Design review of the part built by this model. Coordinates are the model's own, in mm. Coordinates: 2 decimals unless noted, no trailing zeros. Loops run counter-clockwise (first coordinate to the right, second up) from the corner with the lowest first, then second, coordinate; pieces in that order, holes last. Notation, with made-up numbers: (36.25, 86) -> (46.25, 86) arc R15 cw to (46.25, 91) -> close; hole circle Ø2 at (10, -37.5). An arc over 180 degrees is marked (long way). Answer in a Markdown table with one row per item.
Autodesk Fusion 360 part; units mm, degrees
sketch "Front" plane through (0, 0, 0) normal (0, 1, 0) x (1, 0, 0)
  line L0 (-15, -120) -> (15, -120)
  line L1 (15, -120) -> (15, 120)
  line L2 (15, 120) -> (-15, 120)
  line L3 (-15, 120) -> (-15, -120)
  line L4 (0, -120) -> (0, 120) construction
  circle A0 centre (0, -100) radius 4
  circle A1 centre (0, -70) radius 4
  circle A2 centre (0, 50) radius 4
  circle A3 centre (0, 70) radius 4
  circle A4 centre (0, -100) radius 7.5
  circle A5 centre (0, 70) radius 7.5
  dimension "d1" = 240
  dimension "d2" = 30
  dimension "d3" = 8
  dimension "d4" = 8
  dimension "d5" = 8
  dimension "d6" = 8
  dimension "d7" = 50
  dimension "d8" = 20
  dimension "d9" = 30
  dimension "d10" = 20
  dimension "d15" = 15
  dimension "d16" = 15
extrude "Extrude3" add sketch "Front" against normal blind 10 contours A4 | A5 makes body 1 at (7.4907, -6.6667, 100.3738) makes body 2 at (7.4907, -6.6667, -69.6262)
extrude "Extrude4" add sketch "Front" against normal blind 18 contours L0 L1 L2 L3 bodies 1 2
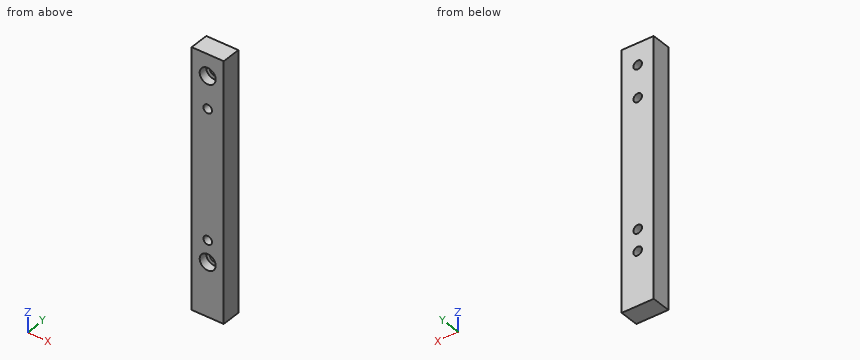
(1) Take a section at C-C on y = -8. Give the boundary of the cut face in (x, z).
Evaluation:
| item | result |
|---|---|
| outline | (-15, -120) -> (15, -120) -> (15, 120) -> (-15, 120) -> close; hole circle Ø8 at (0, -70); hole circle Ø8 at (0, -50); hole circle Ø8 at (0, 70); hole circle Ø8 at (0, 100) |
(2) For pin 1 (9 mm diameter, centred on x = 0, z = -70, fed in from -Y), flat-tipped, find the tip position at first contact; note if it passes through.
Evaluation:
| item | result |
|---|---|
| pin 1 | stops at y = -10 |
(3) Take a section at A-A on z = -50. Give the boundary of the cut face in (x, y).
Evaluation:
| item | result |
|---|---|
| outline | (-15, -18) -> (-4, -18) -> (-4, 0) -> (-15, 0) -> close; (4, -18) -> (15, -18) -> (15, 0) -> (4, 0) -> close |
(4) To check wall thickness, follow probe 1 along Z at (x, y) = (0, -1.75); probe 2 along X at (y, z) = (-6.5, -70); probe 3 along Z at (x, y) = (0, -11.5). State the ranges of each line that lie inside material, in increasing order.
Evaluation:
| item | result |
|---|---|
| probe 1 | z = -120 to -74, -66 to -54, -46 to 66, 74 to 96, 104 to 120 |
| probe 2 | x = -15 to -4, 4 to 15 |
| probe 3 | z = -120 to -77.5, -62.5 to -54, -46 to 66, 74 to 92.5, 107.5 to 120 |
(5) Take a section at B-B on x = 0. Give the boundary of the cut face in (y, z).
Evaluation:
| item | result |
|---|---|
| outline | (-18, -120) -> (0, -120) -> (0, -74) -> (-10, -74) -> (-10, -77.5) -> (-18, -77.5) -> close; (-18, -62.5) -> (-10, -62.5) -> (-10, -66) -> (0, -66) -> (0, -54) -> (-18, -54) -> close; (-18, -46) -> (0, -46) -> (0, 66) -> (-18, 66) -> close; (-18, 74) -> (0, 74) -> (0, 96) -> (-10, 96) -> (-10, 92.5) -> (-18, 92.5) -> close; (-18, 107.5) -> (-10, 107.5) -> (-10, 104) -> (0, 104) -> (0, 120) -> (-18, 120) -> close |
